Build history of the part. All positions in model axes, mm. Face numbers are marked on the shaded views. A direction names the side the tool comes from. Round coordinates to 2 decimals unless told otherwise and drop trailing zeros. Loops run counter-clockwise (first coordinate to the right, second up) from the corner with the lowest first, then second, coordinate; pieces in that order, holes last. Notation, with made-up numbers: (-22.75, -2) - (24.25, -2) arc R10 ccw to (24.25, 8) - close; hole circle Ø5 at (44.25, 25). An arc over 180 degrees is marked (long way). Use a Markdown table: item, result.
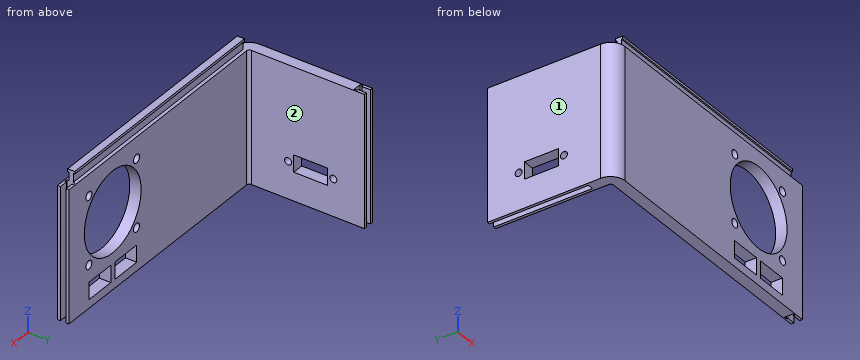
from build123d import *

# Parameters (mm, degrees)
PAD_DEPTH       = 46.5
SKETCH114_W     = 3
SKETCH114_H     = 2
SKETCH114_W_2   = 1
SKETCH114_H_2   = 3
POCKET_DEPTH    = 46.501
SKETCH116_R     = 14.23
SKETCH116_R_2   = 1.5
POCKET001_DEPTH = 5
SKETCH_W        = 2
SKETCH_H        = 35
POCKET002_DEPTH = 7
POCKET003_START = 7
SKETCH117_W     = 2
SKETCH117_H     = 3
SKETCH117_W_2   = 3
SKETCH117_H_2   = 1
POCKET003_DEPTH = 40
PAD001_START    = -4
SKETCH119_W     = 1.5
SKETCH119_H     = 3
SKETCH119_W_2   = 2.5
SKETCH119_H_2   = 0.9
PAD001_DEPTH    = 85
SKETCH118_R     = 1.25
SKETCH118_W     = 12
SKETCH118_H     = 6
POCKET004_DEPTH = 94.001
SKETCH120_W     = 11
SKETCH120_H     = 6
POCKET005_DEPTH = 5


with BuildPart() as part:
    # Sketch112 → Pad (new body)
    with BuildSketch(Plane.XY):
        with BuildLine():
            Line((0, 0), (-89, 0))
            ThreePointArc((-94, 5), (-92.535534, 1.464466), (-89, 0))
            Line((-94, 5), (-94, 45))
            Line((-94, 45), (-90, 45))
            Line((-90, 5), (-90, 45))
            ThreePointArc((-90, 5), (-89.707107, 4.292893), (-89, 4))
            Line((0, 4), (-89, 4))
            Line((0, 4), (0, 0))
        make_face()
    extrude(amount=PAD_DEPTH)

    # Sketch114 → Pocket (cut, through all)
    with BuildSketch(Plane.XY):
        with Locations((-1.5, 2)):
            Rectangle(SKETCH114_W, SKETCH114_H)
        with Locations((-3.5, 2)):
            Rectangle(SKETCH114_W_2, SKETCH114_H_2)
    extrude(amount=POCKET_DEPTH, mode=Mode.SUBTRACT)

    # Sketch116 → Pocket001 (cut)
    with BuildSketch(Plane.XZ):
        with Locations((-21.95, 27)):
            Circle(SKETCH116_R)
        with Locations((-10, 38.95)):
            Circle(SKETCH116_R_2)
        with Locations((-33.9, 38.95)):
            Circle(SKETCH116_R_2)
        with Locations((-33.9, 15.05)):
            Circle(SKETCH116_R_2)
        with Locations((-10, 15.05)):
            Circle(SKETCH116_R_2)
    extrude(amount=-POCKET001_DEPTH, mode=Mode.SUBTRACT)

    # Sketch → Pocket002 (cut)
    with BuildSketch(Plane.XY):
        with Locations((-92, 27.5)):
            Rectangle(SKETCH_W, SKETCH_H)
    extrude(amount=POCKET002_DEPTH, mode=Mode.SUBTRACT)

    # Sketch117 → Pocket003 (cut)
    with BuildSketch(Plane.XY.offset(POCKET003_START)):
        with Locations((-92, 43.5)):
            Rectangle(SKETCH117_W, SKETCH117_H)
        with Locations((-92, 41.5)):
            Rectangle(SKETCH117_W_2, SKETCH117_H_2)
    extrude(amount=POCKET003_DEPTH, mode=Mode.SUBTRACT)

    # Sketch119 → Pad001 (join)
    with BuildSketch(Plane.YZ.offset(PAD001_START)):
        with Locations((2, 48)):
            Rectangle(SKETCH119_W, SKETCH119_H)
        with Locations((2, 49.95)):
            Rectangle(SKETCH119_W_2, SKETCH119_H_2)
    extrude(amount=-PAD001_DEPTH)

    # Sketch118 → Pocket004 (cut, through all)
    with BuildSketch(Plane.YZ):
        with Locations((34, 13)):
            Circle(SKETCH118_R)
        with Locations((18, 13)):
            Circle(SKETCH118_R)
        with Locations((26, 13)):
            Rectangle(SKETCH118_W, SKETCH118_H)
    extrude(amount=-POCKET004_DEPTH, mode=Mode.SUBTRACT)

    # Sketch120 → Pocket005 (cut)
    with BuildSketch(Plane.XZ):
        with Locations((-15.5, 6)):
            Rectangle(SKETCH120_W, SKETCH120_H)
        with Locations((-28.5, 6)):
            Rectangle(SKETCH120_W, SKETCH120_H)
    extrude(amount=-POCKET005_DEPTH, mode=Mode.SUBTRACT)


solid = part.part
Q1. Drop flat-ended pins along their axis: pin 1 (1.2 mm diameter, centred on x = -91.5, y = 26.5, fed in from +Z); pin 2 (12 mm diameter, centred on x = -57.5, y = 11, fed in from +Z); pin 3 (2 mm diameter, centred on y = 24.5, z = 31.5, fed in from +X); pin 4 (4.5 mm diameter, centred on x = -92, z = 11.5, fed in from -Y). Give the stop position or say it passes through.
Results found:
| item | result |
|---|---|
| pin 1 | stops at z = 46.5 |
| pin 2 | passes through |
| pin 3 | stops at x = -90 |
| pin 4 | stops at y = 0.06 |
Q2. Cut at A-A, the plane x = -21.95. List the corners of the cut face in (y, z), plus the area to 3 significant figures.
Results found:
| item | result |
|---|---|
| outline | (0, 0) - (4, 0) - (4, 12.77) - (0, 12.77) - close; (0, 41.23) - (4, 41.23) - (4, 46.5) - (2.75, 46.5) - (2.75, 49.5) - (3.25, 49.5) - (3.25, 50.4) - (0.75, 50.4) - (0.75, 49.5) - (1.25, 49.5) - (1.25, 46.5) - (0, 46.5) - close |
| area | 78.9 mm2 |
Q3. Cut at D-D, the plane x = -80. List the corners of the cut face in (y, z), plus the area to 3 significant figures.
Results found:
| item | result |
|---|---|
| outline | (0, 0) - (4, 0) - (4, 46.5) - (2.75, 46.5) - (2.75, 49.5) - (3.25, 49.5) - (3.25, 50.4) - (0.75, 50.4) - (0.75, 49.5) - (1.25, 49.5) - (1.25, 46.5) - (0, 46.5) - close |
| area | 193 mm2 |
Q4. Which spindle directions (+Z, -Z, +X, -X, +Y, -Y) get a long thin tool onto all of the face, cutting with end or side? Do the marked faces 1 and 2. Say none if no direction does.
Results found:
| item | result |
|---|---|
| face 1 | +Z, -Z, -X, +Y, -Y |
| face 2 | +Z, -Z, +X, +Y |
Q5. Cut at C-C, the plane z = 28. List the corners of the cut face in (x, y).
Results found:
| item | result |
|---|---|
| outline | (-94, 5) arc R5 ccw to (-89, 0) - (-36.14, 0) - (-36.14, 4) - (-89, 4) arc R1 cw to (-90, 5) - (-90, 45) - (-91, 45) - (-91, 42) - (-90.5, 42) - (-90.5, 41) - (-93.5, 41) - (-93.5, 42) - (-93, 42) - (-93, 45) - (-94, 45) - close; (-7.76, 0) - (0, 0) - (0, 1) - (-3, 1) - (-3, 0.5) - (-4, 0.5) - (-4, 3.5) - (-3, 3.5) - (-3, 3) - (0, 3) - (0, 4) - (-7.76, 4) - close |
Q6. Cut at B-B, the plane y = 34. List the corners of the cut face in (x, z), plus the area to 3 significant figures.
Results found:
| item | result |
|---|---|
| outline | (-94, 0) - (-93, 0) - (-93, 7) - (-91, 7) - (-91, 0) - (-90, 0) - (-90, 11.75) - (-94, 11.75) - close; (-94, 14.25) - (-90, 14.25) - (-90, 46.5) - (-94, 46.5) - close |
| area | 162 mm2 |
Q7. Probe line 1 (X direction, y = 2, z = 38); line 2 (Z direction, x = -91.2, y = 34); line 3 (X direction, y = 41.5, z = 30). List the from-to ranges inside material, lowest first.
Results found:
| item | result |
|---|---|
| line 1 | x = -93 to -35.06, -32.74 to -30.98, -12.92 to -11.16, -8.84 to -4 |
| line 2 | z = 7 to 11.75, 14.25 to 46.5 |
| line 3 | x = -94 to -93.5, -90.5 to -90 |
